Verification items for the finished model (mm, model axes). Round coordinates to 2 decimals unless told otherwise and drop trailing zeros. Order: outer loops, then holes, each group sorted by start corner. A loop starts at its lowest first (then second) coordinate and runs counter-clockwise, first axis right, second up. Notation, with made-up numbers: (71, -11.75) -> (90, -11.75) arc R20 cw to (90, 5.25) -> close; hole circle Ø1 at (-10.5, 73). An arc over 180 degrees is marked (long way). Return JSON: item names as keys, results as strings. Group by question number.
1) Section check C-C on z = 9. Enter the section's corners in (x, y).
2) Depth check by flat-ended pin: pin 1 (8 mm diameter, centred on x = 25.5, y = 0.5, fed in from +Z); pin 2 (6 mm diameter, centred on x = 5.5, z = 8, fed in from -Y); pin 3 (3 mm diameter, centred on y = 22.5, z = 8, fed in from -X). Enter the tip coordinate at first touch or a pass-through.
3) Scan lines: L1, parallel to Y at x = 0, z = 9.5; L2, parallel to Y at x = 0, z = 1.25; L3, parallel to X at y = -17, z = 8. Record each from-to range of solid material in increasing order.
4) Section check D-D on y = -17. Enter the section's corners in (x, z), plus the area to 3 significant figures.
5) Section check A-A on y = 0. Enter the section's corners in (x, z).
6) Section check B-B on x = -23. Enter the section's corners in (y, z).
Autodesk Fusion 360 part; units mm, degrees
sketch "Sketch2" plane through (0, 0, 0) normal (0, 0, 1) x (1, 0, 0)
  circle A0 centre (0, 0) radius 34
  circle A1 centre (0, 0) radius 22.5
  circle A2 centre (0, 34) radius 2.15
  circle A3 centre (0, 34) radius 4.15
  circle A4 centre (-29.4449, -17) radius 2.15
  circle A5 centre (29.4449, -17) radius 2.15
  circle A6 centre (0, 0) radius 30.5
  line L0 (0, 38.15) -> (0, 29.85) construction
  line L1 (4.15, 38.15) -> (-4.15, 29.85) construction
  line L2 (-4.15, 38.15) -> (4.15, 29.85) construction
  circle A7 centre (-29.4449, -17) radius 4.15
  circle A8 centre (29.4449, -17) radius 4.15
  point P0 (0, 34)
  dimension "d19" = 68
  dimension "d21" = 45
  dimension "d22" = 4.3
  dimension "d23" = 2
  dimension "d25" = 360
  dimension "d29" = 61
extrude "main" add sketch "Sketch2" along normal blind 10 contours A0 A3 A6 A8 | A0 A2 A3 A6 | A0 A2 A3 | A0 A5 A8 | A0 A5 A6 A8 | A0 A3 A6 A7 | A0 A6 A7 A8 | A0 A4 A6 A7 | A0 A4 A7
ref_plane "WorkPlane1" through (-4.15, 34, 6.304) normal (-1, 0, 0) x (0, 1, 0)
sketch "Sketch3" plane through (-4.15, 0, 0) normal (-1, 0, 0) x (0, -1, 0)
  line L0 (-33.7467, 0) -> (-39.4074, 5.6606)
  line L1 (-33.7467, 0) -> (-41.6458, 0) construction
  line L2 (-33.7467, 0) -> (-39, 0)
  line L3 (-33.7467, 0) -> (-39.699, 0)
  line L4 (-39.4074, 5.6606) -> (-39.4074, 0)
  line L5 (13.2861, 0) -> (-33.7467, 0)
  line L6 (13.2861, 0) -> (13.2861, 10)
  line L7 (13.2861, 10) -> (-33.7467, 10)
  line L8 (-33.7467, 10) -> (-33.7467, 0)
  dimension "d43" = 45
extrude "side cut" cut sketch "Sketch3" against normal blind 15 contours L0 L2 L3 L4
pattern_circular "C-Pattern1" count 3 over 360 about axis through (0, 0, 1.75) along (0, 0, 1) of "side cut"
equation "gear_width = 10 mm"
equation "gear_backlash = 0.25 mm"
equation "gear_sp = ( ( gear_Ns + gear_Np ) / 2 ) * 1 mm"
equation "gear_OD = ( gear_Nr ) * 1 mm + 8 mm"
equation "ring_width = 52 mm"
equation "m3_hole_thickness = 2 mm"
equation "m3_inserts = 4.3 mm"
equation "d19 = gear_OD"
equation "output_bearing_od = 47 mm"
equation "d21 = output_bearing_od - 2 mm"
equation "d22 = m3_inserts"
equation "d23 = m3_hole_thickness"
equation "d29 = gear_OD - wall_thickness"
equation "wall_thickness = 7 mm"
equation "d33 = height"
equation "height = 10 mm"
Check result:
{
 "1": {"outline": "(-31.3, -13.29) arc R4.15 ccw (long way) to (-27.15, -20.46) arc R34 ccw to (27.15, -20.46) arc R4.15 ccw (long way) to (31.3, -13.29) arc R34 ccw to (4.14, 33.75) arc R4.15 ccw (long way) to (-4.14, 33.75) arc R34 ccw to start; hole circle Ø4.3 at (-29.44, -17); hole circle Ø61 at (0, 0); hole circle Ø4.3 at (0, 34); hole circle Ø4.3 at (29.44, -17)"},
 "2": {"pin 1": "through", "pin 2": "y = -33.91", "pin 3": "x = -26.74"},
 "3": {"L1": "-34 to -30.5, 30.5 to 31.85, 36.15 to 38.15", "L2": "-34 to -30.5, 30.5 to 31.85", "L3": "-33.59 to -31.59, -27.29 to -25.32, 25.32 to 27.29, 31.59 to 33.59"},
 "4": {"outline": "(-33.59, 3.85) -> (-31.59, 2.12) -> (-31.59, 10) -> (-33.59, 10) -> close; (-27.29, 0) -> (-25.32, 0) -> (-25.32, 10) -> (-27.29, 10) -> close; (25.32, 0) -> (27.29, 0) -> (27.29, 10) -> (25.32, 10) -> close; (31.59, 2.12) -> (33.59, 3.85) -> (33.59, 10) -> (31.59, 10) -> close", "area": "67.5 mm^2"},
 "5": {"outline": "(-34, 0) -> (-30.5, 0) -> (-30.5, 10) -> (-34, 10) -> close; (30.5, 0) -> (34, 0) -> (34, 10) -> (30.5, 10) -> close"},
 "6": {"outline": "(-25.04, 0) -> (-20.03, 0) -> (-20.03, 10) -> (-25.04, 10) -> close; (20.03, 0) -> (25.04, 0) -> (25.04, 10) -> (20.03, 10) -> close"}
}
